from build123d import *

# Parameters (mm, degrees)
F0_W     = 100.517206
F0_H     = 81.81633
F1_DEPTH = 30.48
F2_R     = 32.949499
F2_R_2   = 27.533167
F3_DEPTH = 25.4


with BuildPart() as f1:
    # F0 (on Front) → F1 (new body)
    with BuildSketch(Plane.XZ):
        Rectangle(F0_W, F0_H)
    extrude(amount=F1_DEPTH)

    # F2 (on Front) → F3 (join)
    with BuildSketch(Plane.XZ):
        Circle(F2_R)
        Circle(F2_R_2, mode=Mode.SUBTRACT)
    extrude(amount=-F3_DEPTH)


solid = f1.part
Geometry: final body of the model. Coordinates: model frame, mm. A direction names the side the tool comes from. Round coordinates to 2 decimals unless told otherwise and drop trailing zeros. Loops run counter-clockwise (first coordinate to the right, second up) from the corner with the lowest first, then second, coordinate; pieces in that order, holes last.
Q1. Section A-A on z = 0. Return loops of the section in (x, y), plus the area to 3 significant figures.
Q2. Pull-direction query (X, two-part tool) for faces 3 (the flat face through (-50.259, -15, -1)), 4 (the flat face through (0, 0, 0)), 5 (the flat face through (-1, -15, -40.908)); classes: released by +X, released by -X, zero draft, split by the parting line, or undercut.
Q3. Material intervals for L1, parallel to Z at x = 0, y = 6.5; L2, parallel to X at y = 11, z = 1 (3 decimals); L3, parallel to Y at x = -16, z = -4, sorted ascending.
Q4. Section B-B on x = 0. Return loops of the section in (y, z), plus the area to 3 significant figures.
Q5. Pin query (flat end, axial travel): P1, Ø4, axis at y = 6.5, z = 11.5, coming from the +X side; P2, Ø1, axis at y = 17.5, z = 16, coming from the -X side; P3, Ø1, axis at x = -34, z = 13, coming from the +Y side. Return the tip coordinate at first contact, or that it passes through.
Q6. Access query for faces 1 (the flat face through (50.259, -15, -1)), 2 (the cylindrical face through (-5.97, 12.52, -26.88)). Directions: +Z, -Z, +X, -X, +Y, -Y. A direction counts if a zero-diameter tool reaches every point of the face in a straight line with its end or side. Return the directions, or none.
Q7. Section C-C on y = 15.5. Return loops of the section in (x, z), plus the area to 3 significant figures.
Q8. Section D-D on z = -29. Return loops of the section in (x, y), plus the area to 3 significant figures.
Evaluation:
1. outline: (-50.26, -30.48) - (50.26, -30.48) - (50.26, 0) - (32.95, 0) - (32.95, 25.4) - (27.53, 25.4) - (27.53, 0) - (-27.53, 0) - (-27.53, 25.4) - (-32.95, 25.4) - (-32.95, 0) - (-50.26, 0) - close
1. area: 3,340 mm2
2. face 3: released by -X
2. face 4: undercut
2. face 5: zero draft
3. L1: z = -32.95 to -27.53, 27.53 to 32.95
3. L2: x = -32.934 to -27.515, 27.515 to 32.934
3. L3: y = -30.48 to 0
4. outline: (-30.48, -40.91) - (0, -40.91) - (0, -32.95) - (25.4, -32.95) - (25.4, -27.53) - (0, -27.53) - (0, 27.53) - (25.4, 27.53) - (25.4, 32.95) - (0, 32.95) - (0, 40.91) - (-30.48, 40.91) - close
4. area: 2,770 mm2
5. P1: stops at x = 31.55
5. P2: stops at x = -29.08
5. P3: stops at y = 0
6. face 1: +Z, -Z, +X, +Y, -Y
6. face 2: +Y
7. outline: circle Ø65.9 at (0, 0); hole circle Ø55.07 at (0, 0)
7. area: 1,030 mm2
8. outline: (-50.26, -30.48) - (50.26, -30.48) - (50.26, 0) - (15.64, 0) - (15.64, 25.4) - (-15.64, 25.4) - (-15.64, 0) - (-50.26, 0) - close
8. area: 3,860 mm2
